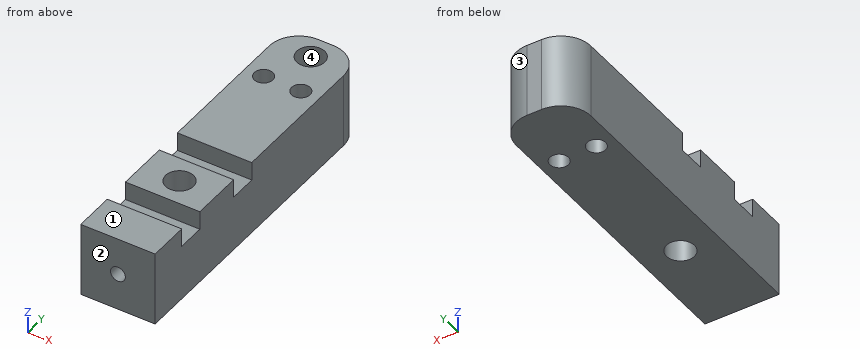
from build123d import *

# Parameters (mm, degrees)
SKETCH2_W           = 25.4
SKETCH2_H           = 109.22
BOSS_EXTRUDE1_DEPTH = 25.4
SKETCH3_R           = 4.7625
SKETCH3_R_2         = 3.175
CUT_EXTRUDE1_DEPTH  = 25.4
SKETCH4_W           = 25.4
SKETCH4_H           = 9.525
CUT_EXTRUDE2_DEPTH  = 6.35
SKETCH5_R           = 4.7625
CUT_EXTRUDE3_DEPTH  = 16.51
SKETCH6_R           = 2.54
CUT_EXTRUDE4_DEPTH  = 17.78
FILLET1_R           = 10.16


with BuildPart() as part:
    # Sketch2 → Boss-Extrude1 (new body)
    with BuildSketch(Plane.XY):
        Rectangle(SKETCH2_W, SKETCH2_H)
    extrude(amount=BOSS_EXTRUDE1_DEPTH)

    # Sketch3 → Cut-Extrude1 (cut)
    with BuildSketch(Plane.XY.offset(25.4)):
        with Locations((0, -22.225)):
            Circle(SKETCH3_R)
        with Locations((6.35, 31.75)):
            Circle(SKETCH3_R_2)
        with Locations((-6.35, 31.75)):
            Circle(SKETCH3_R_2)
    extrude(amount=-CUT_EXTRUDE1_DEPTH, mode=Mode.SUBTRACT)

    # Sketch4 → Cut-Extrude2 (cut)
    with BuildSketch(Plane.XY.offset(25.4)):
        with Locations((0, -8.5725)):
            Rectangle(SKETCH4_W, SKETCH4_H)
        with Locations((0, -35.8775)):
            Rectangle(SKETCH4_W, SKETCH4_H)
    extrude(amount=-CUT_EXTRUDE2_DEPTH, mode=Mode.SUBTRACT)

    # Sketch5 → Cut-Extrude3 (cut)
    with BuildSketch(Plane.XY.offset(25.4)):
        with Locations((0, 46.736)):
            Circle(SKETCH5_R)
    extrude(amount=-CUT_EXTRUDE3_DEPTH, mode=Mode.SUBTRACT)

    # Sketch6 → Cut-Extrude4 (cut)
    with BuildSketch(Plane.XZ.offset(54.61)):
        with Locations((0, 12.7)):
            Circle(SKETCH6_R)
    extrude(amount=-CUT_EXTRUDE4_DEPTH, mode=Mode.SUBTRACT)

    # Fillet1
    fillet1_edges = [part.edges().sort_by_distance(p)[0] for p in [
        (-12.7, 54.61, 12.7),
        (12.7, 54.61, 12.7),
    ]]
    fillet(fillet1_edges, radius=FILLET1_R)


solid = part.part
Can you work these out from the model? Positions are in its coordinate system, mm. Face numbers are marked on the shaded views. Round coordinates to 2 decimals unless told otherwise and drop trailing zeros. Loops run counter-clockwise (first coordinate to the right, second up) from the corner with the lowest first, then second, coordinate; pieces in that order, holes last. Notation, with made-up numbers: (53, 9) - (109, 9) arc R32 ccw to (109, 36) - close; hole circle Ø3 at (86.5, -5.5). An arc over 180 degrees is marked (long way). Answer in a Markdown table with one row per item. Add a question column.
Q1. I need wall thicknesses on L1, parallel to Y at x = 0, z = 17; L2, parallel to Y at x = 0, z = 19.25 (1 decimal); L3, parallel to Y at x = 0, z = 10.5. Which ranges of each line are inside material? Lowest first, please.
Q2. I want a section at D-D on y = -46. List the corners of the cut face in (x, z) for me.
Q3. We'd pull the mould along Y, two halves only. Please class the marked faces 1, 2, 3 and 4: pulls with the +Y half, pulls with the -Y half, needs draft (parallel to the pull), parting line crosses it, or undercut.
Q4. I want a section at B-B on y = -19.5. List the corners of the cut face in (x, z) for me.
Q5. I want a section at C-C on z = 12.7. Count the separate pieces of the cut face and the enclosed holes in it, and give its area (3 significant figures).
Q6. For pin 1 Ø8.5 at (x, y) = (0, 46.736) entering from -Z; pin 2 Ø4 at (x, y) = (-6.35, 31.75) entering from +Z; pin 3 Ø3 at (x, y) = (5, -7) entering from +Z; pin 4 Ø5 at (x, z) = (-5.5, 21.5) entering from +Y, each with a flat end and sliding along its axis, tell me the tip position at first contact or that it passes through.
A:
| question | item | result |
|---|---|---|
| 1 | L1 | -54.61 to -26.99, -17.46 to 41.97, 51.5 to 54.61 |
| 1 | L2 | -54.6 to -40.6, -31.1 to -27, -17.5 to -13.3, -3.8 to 42, 51.5 to 54.6 |
| 1 | L3 | -36.83 to -26.99, -17.46 to 41.97, 51.5 to 54.61 |
| 2 | outline | (-12.7, 0) - (12.7, 0) - (12.7, 25.4) - (-12.7, 25.4) - close; hole circle Ø5.08 at (0, 12.7) |
| 3 | face 1 | needs draft |
| 3 | face 2 | pulls with the -Y half |
| 3 | face 3 | pulls with the +Y half |
| 3 | face 4 | undercut |
| 4 | outline | (-12.7, 0) - (-3.91, 0) - (-3.91, 25.4) - (-12.7, 25.4) - close; (3.91, 0) - (12.7, 0) - (12.7, 25.4) - (3.91, 25.4) - close |
| 5 | separate pieces | 1 |
| 5 | enclosed holes | 4 |
| 5 | area | 2,430 mm^2 |
| 6 | pin 1 | z = 0 |
| 6 | pin 2 | through |
| 6 | pin 3 | z = 19.05 |
| 6 | pin 4 | y = 54.6 |
